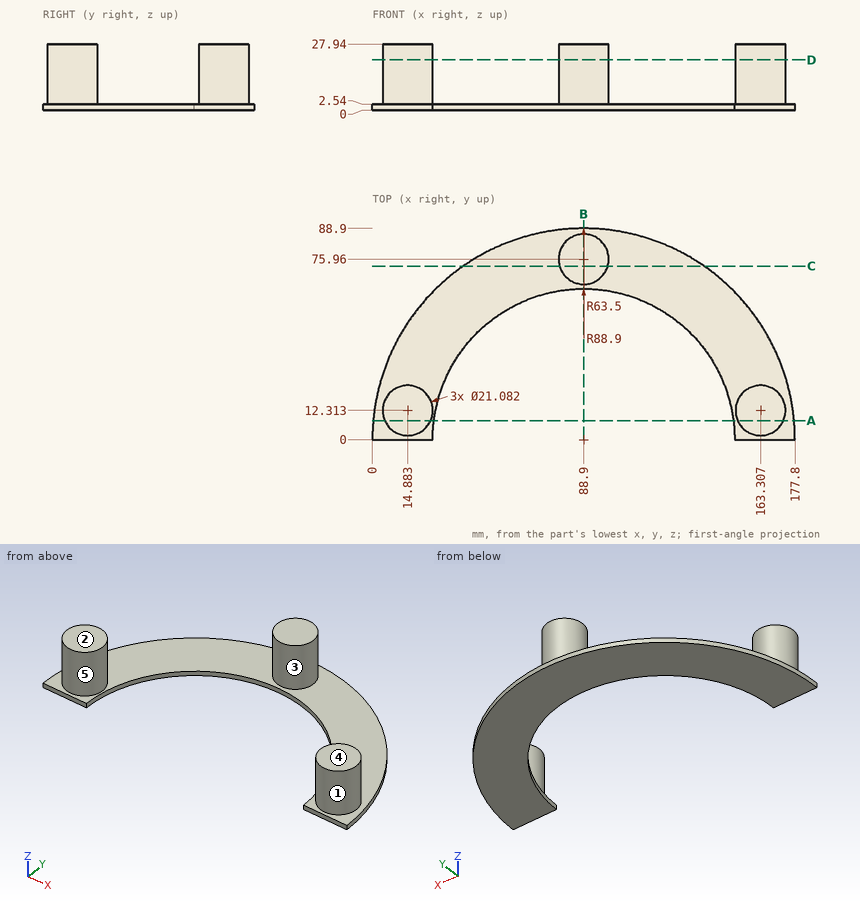
For this review, use the dimensioned drawing (mm, ordinates from the lowest corner) and the shaded views. A direction names the side the tool comes from. Coordinates: 2 decimals unless noted, no trailing zeros. Order: outer loops, then holes, each group sorted by start corner. A loop starts at its lowest first (then second) coordinate and runs counter-clockwise, first axis right, second up. Notation, with made-up numbers: (25, -7.5) - (70, -7.5) arc R8 ccw to (70, -3.5) - close; hole circle Ø1 at (21, -8). An arc over 180 degrees is marked (long way). Use one line per item in the form item = value.
Q1. Consider section B-B (x = 88.9). Give the boundary of the cut face in (y, z), then the cut area to 3 significant figures.
Checked values:
outline = (63.5, 0) - (88.9, 0) - (88.9, 2.54) - (86.5, 2.54) - (86.5, 27.94) - (65.42, 27.94) - (65.42, 2.54) - (63.5, 2.54) - close
area = 600 mm2
Q2. For the marked faces 1 and 2, list the 3-axis set-ups (+Z, -Z, +X, -X, +Y, -Y) from which the entire face can be reached by the end or side of a thin tool; tool diameter is ignored.
Checked values:
face_1 = +Z
face_2 = +Z, +X, -X, +Y, -Y
Q3. For P1, Ø8, axis at y = 36.5, z = 7, coming from the -X side; P2, Ø10, axis at y = 79.5, z = 23, coming from the -X side, all flat-tipped, find the tip position at first contact; note any pin that passes through.
Checked values:
P1 = through
P2 = 78.36
Q4. For probe 1 along Z at (x, y) = (147, 49.5); probe 2 along X at (y, z) = (6.5, 8.25) (1 decimal); probe 3 along X at (y, z) = (11, 3.75) (1 decimal), list the stretches that pass through material, from the lowest coordinate up. Write a range as from..to.
Checked values:
probe_1 = 0..2.54
probe_2 = 6.1..23.7, 154.5..172.1
probe_3 = 4.4..25.3, 152.8..173.8
Q5. Consider section D-D (z = 21.25). Give the boundary of the cut face in (x, y) (1 decimal).
Checked values:
outline = circle Ø21.1 at (14.9, 12.3); circle Ø21.1 at (88.9, 76); circle Ø21.1 at (163.3, 12.3)
Q6. Consider section C-C (y = 73). Give the boundary of the cut face in (x, z).
Checked values:
outline = (38.16, 0) - (139.64, 0) - (139.64, 2.54) - (99.02, 2.54) - (99.02, 27.94) - (78.78, 27.94) - (78.78, 2.54) - (38.16, 2.54) - close
Q7. Draft analysis for pull direction X (two halves, no side actions). For the marked faces 3, 4 and 5, state which applies: +X half, -X half, draft (parallel to the pull), parting line (faces both ways), or undercut.
Checked values:
face_3 = parting line
face_4 = draft
face_5 = undercut
Q8. Consider section A-A (y = 8). Give the boundary of the cut face in (x, z) (1 decimal).
Checked values:
outline = (0.4, 0) - (25.9, 0) - (25.9, 2.5) - (24.5, 2.5) - (24.5, 27.9) - (5.3, 27.9) - (5.3, 2.5) - (0.4, 2.5) - close; (151.9, 0) - (177.4, 0) - (177.4, 2.5) - (172.9, 2.5) - (172.9, 27.9) - (153.7, 27.9) - (153.7, 2.5) - (151.9, 2.5) - close
